Can you work these out from the model? Positions are in its coordinate system, mm. A direction names the side the tool comes from. Give positions to 0.01 mm unless a question says otherwise; leave off trailing zeros. Order: outer loops, then holes, each group sorted by start corner. A loop starts at its lowest first (then second) coordinate and runs counter-clockwise, first axis right, second up. Notation, with made-up numbers: (28, 43) -> (61, 43) arc R18 ccw to (61, 48) -> close; hole circle Ø3 at (16, 87). An arc over 180 degrees is marked (long way). Answer as CSV lines item,"result".
```python
from build123d import *

# Parameters (mm, degrees)
SKETCH1_R           = 2.159
SKETCH1_W           = 6.35
SKETCH1_H           = 6.35
SKETCH1_H_2         = 3.81
BOSS_EXTRUDE1_DEPTH = 6.35


with BuildPart() as part:
    # Sketch1 → Boss-Extrude1 (new body)
    with BuildSketch(Plane(origin=(0, 0, 0), x_dir=(1, 0, 0), z_dir=(0, 1, 0))):
        Polygon((-41.148, -17.907), (41.148, -17.907), (41.148, 17.907), (28.702, 17.907), (28.702, 11.049), (-28.702, 11.049), (-28.702, 17.907), (-41.148, 17.907), align=None)
        with Locations(Location((34.925, 0, 0), (0, 0, 270))):
            Circle(SKETCH1_R, mode=Mode.SUBTRACT)
        with Locations((-34.925, 0)):
            Circle(SKETCH1_R, mode=Mode.SUBTRACT)
        with Locations((0, -11.684)):
            Rectangle(SKETCH1_W, SKETCH1_H, mode=Mode.SUBTRACT)
        with Locations((0, 6.096)):
            Rectangle(SKETCH1_W, SKETCH1_H_2, mode=Mode.SUBTRACT)
        with Locations((34.925, 11.684)):
            Rectangle(SKETCH1_W, SKETCH1_H, mode=Mode.SUBTRACT)
        with Locations((34.925, -11.684)):
            Rectangle(SKETCH1_W, SKETCH1_H, mode=Mode.SUBTRACT)
        with Locations((-34.925, 11.684)):
            Rectangle(SKETCH1_W, SKETCH1_H, mode=Mode.SUBTRACT)
        with Locations((-34.925, -11.684)):
            Rectangle(SKETCH1_W, SKETCH1_H, mode=Mode.SUBTRACT)
    extrude(amount=BOSS_EXTRUDE1_DEPTH)


solid = part.part
```
Item 1: Imagine slicing it at C-C, the plane y = 4.25. Give the number of separate pieces and of enclosed holes in the cut face, then the cut area to 3 significant figures.
Numbers:
separate pieces,"1"
enclosed holes,"8"
area,"2,300 mm²"
Item 2: Imagine slicing it at B-B, the plane z = 0. Please give me the cut outline in (x, y), then the cut area to 3 significant figures.
Numbers:
outline,"(-41.15, 0) -> (-37.08, 0) -> (-37.08, 6.35) -> (-41.15, 6.35) -> close; (-32.77, 0) -> (32.77, 0) -> (32.77, 6.35) -> (-32.77, 6.35) -> close; (37.08, 0) -> (41.15, 0) -> (41.15, 6.35) -> (37.08, 6.35) -> close"
area,"468 mm²"
Item 3: Please list where these lines run through material, in increasing order: line 1 along Z through (x, y) = (-1.5, 5.75); line 2 along X through (y, z) = (0.5, 9.5) (3 decimals); line 3 along X through (y, z) = (3.5, 0).
Numbers:
line 1,"z = -11.05 to -8, -4.19 to 8.51, 14.86 to 17.91"
line 2,"x = -41.148 to -38.1, -31.75 to -3.175, 3.175 to 31.75, 38.1 to 41.148"
line 3,"x = -41.15 to -37.08, -32.77 to 32.77, 37.08 to 41.15"
Item 4: For faces 1 (the flat face through (35, 3, -17.907)), 2 (the flat face through (-35, 3, 14.859)), which set-ups out of +Z, -Z, +X, -X, +Y, -Y let a thin tool reach every point of the face, with its end or its side?
Numbers:
face 1,"-Z, +X, -X, +Y, -Y"
face 2,"+Y, -Y"
Item 5: For pin 1 (1.9 mm diameter, centred on x = 4, y = 2.5, fed in from -Z), with a flat end and sliding along its axis, tell me the tip position at first contact or that it passes through.
Numbers:
pin 1,"stops at z = -11.05"
Item 6: We'd pull the mould along Z, two halves only. Please class faces 3 (the flat face through (0, 3, -11.049)), 4 (the flat face through (-41.148, 3, 0)), 5 (the flat face through (-1, 3, 17.907)), 6 (the flat face through (31.75, 3, 12)): released by +Z, released by -Z, zero draft, split by the parting line, or undercut.
Numbers:
face 3,"released by -Z"
face 4,"zero draft"
face 5,"released by +Z"
face 6,"undercut"
Item 7: Imagine slicing it at D-D, the plane x = 17. Please give me the cut outline in (y, z).
Numbers:
outline,"(0, -11.05) -> (6.35, -11.05) -> (6.35, 17.91) -> (0, 17.91) -> close"
Item 8: Imagine slicing it at A-A, the plane z = -13. Please give me the cut outline in (x, y), then the cut area to 3 significant figures.
Numbers:
outline,"(-41.15, 0) -> (-38.1, 0) -> (-38.1, 6.35) -> (-41.15, 6.35) -> close; (-31.75, 0) -> (-28.7, 0) -> (-28.7, 6.35) -> (-31.75, 6.35) -> close; (28.7, 0) -> (31.75, 0) -> (31.75, 6.35) -> (28.7, 6.35) -> close; (38.1, 0) -> (41.15, 0) -> (41.15, 6.35) -> (38.1, 6.35) -> close"
area,"77.4 mm²"
